Input: part model. Units: mm. Frame: model coordinates. A direction names the side the tool comes from. Round coordinates to 2 decimals unless told otherwise and drop trailing zeros. Loops run counter-clockwise (first coordinate to the right, second up) from the corner with the lowest first, then second, coordinate; pieces in that order, holes last. Notation, with made-up numbers: (88.25, 65.25) -> (138.25, 65.25) arc R15 ccw to (138.25, 84.25) -> close; hole circle Ø7 at (53, 44.25). An arc over 180 degrees is marked (long way). One line per question, with ' | ' between items. Start each with the question number.
Q1. Cut plane A-A on x = 4. Return loops of the section in (y, z).
Q2. Contact query for flat-ended pins moving along their axis: P1, Ø1.6, axis at x = 55, y = -18, coming from the -Z side; P2, Ø5, axis at x = 1.5, y = -9, coming from the -Z side; P3, Ø5, axis at x = 63.5, y = -1.5, coming from the +Z side. Output: stop coordinate, or through.
Q3. Cut plane C-C on x = 31. Return loops of the section in (y, z).
Q4. Cut plane D-D on y = 4. Return loops of the section in (x, z).
Q5. Cut plane B-B on x = 65. Return loops of the section in (y, z), and give its area (3 significant figures).
Q6. Material intervals for L1, parallel to Z at x = 80, y = 15.75; L2, parallel to Y at x = 11, z = -10; L3, parallel to Z at x = 48.5, y = 14, sorted ascending.
Q7. Access query for faces 1 (the face through (94, 18, 7)), 2 (the face through (26, 16, -17)), 3 (the face through (90.959, -0.224, -57.393)). Directions: +Z, -Z, +X, -X, +Y, -Y. A direction counts if a zero-diameter tool reaches every point of the face in a straight line with its end or side. Return the directions, or none.
Q8. Mould query, pull axis Y, two halves, no side actions, for faces 4 (the face through (35.9, 12.4, 9)), 5 (the face through (74, 19, 5)), 6 (the face through (93.14, -17.99, -2.1)). Classes: pulls with the +Y half, pulls with the -Y half, needs draft (parallel to the pull), parting line crosses it, or undercut.
from build123d import *

# Parameters (mm, degrees)
F1_DEPTH  = 16
F2_W      = 70
F2_H      = 3
F3_DEPTH  = 2
F4_W      = 50
F4_H      = 14
F5_DEPTH  = 2
F6_R      = 1
F9_DEPTH  = 2
F11_DEPTH = 38.001
F13_D     = 4
F14_R     = 3
F14_R_2   = 2
F15_DEPTH = 5
F16_R     = 3


# Not quite as in the source:
# - a pattern or mirror of a feature is missing from the dataset's text; its kind, count and spacing are read off the source's solid


with BuildPart() as f1:
    # F0 (on Front) → F1 (new body)
    with BuildSketch(Plane.XZ):
        with BuildLine():
            Line((94, 11), (0, 11))
            ThreePointArc((0, 11), (-11, 0), (0, -11))
            Line((0, -11), (19, -11))
            ThreePointArc((19, -11), (21.7681124643, -11.8361612201), (23.6103896104, -14.064978646))
            ThreePointArc((23.6103896104, -14.064978646), (47.9223026847, -44.6255578719), (84.6125434697, -57.9988278946))
            ThreePointArc((84.6125434697, -57.9988278946), (90.1511361286, -59.2227601314), (94.7495356371, -62.543714922))
            Line((94.7495356371, -62.543714922), (96.0448662588, -61))
            ThreePointArc((96.0448662588, -61), (90.8779784788, -57.357163598), (84.7034264019, -56))
            ThreePointArc((84.7034264019, -56), (49.0672193413, -42.9854179344), (25.4545454545, -13.2909701044))
            ThreePointArc((25.4545454545, -13.2909701044), (22.87535745, -10.1706257081), (19, -9))
            Line((19, -9), (0, -9))
            ThreePointArc((0, -9), (-9, 0), (0, 9))
            Line((0, 9), (94, 9))
            Line((94, 9), (94, 11))
        make_face()
    extrude(amount=F1_DEPTH)

    # F2 (on face) → F3 (join)
    with BuildSketch(Plane.XY.offset(11)):
        with Locations((59, -17.5)):
            Rectangle(F2_W, F2_H)
    extrude(amount=-F3_DEPTH)

    # F4 (on face) → F5 (join)
    with BuildSketch(Plane.XZ.offset(19)):
        with Locations((69, 4)):
            Rectangle(F4_W, F4_H)
    extrude(amount=-F5_DEPTH)

    # F6
    f6_edges = [f1.edges().sort_by_distance(p)[0] for p in [
        (59, -19, 11),
    ]]
    fillet(f6_edges, radius=F6_R)

    # F7: F1 across plane


with BuildPart() as f1_1:
    add(f1.part)
    add(f1.part.mirror(Plane.XZ))

    # F8 (on face) → F9 (cut)
    with BuildSketch(Plane.XY.offset(11)):
        with BuildLine():
            Line((94, 12), (34, 12))
            ThreePointArc((34, 12), (22, 0), (34, -12))
            Line((34, -12), (94, -12))
            Line((94, -12), (94, 12))
        make_face()
    extrude(amount=-F9_DEPTH, mode=Mode.SUBTRACT)

    # F10 (on face) → F11 (cut, through all)
    with BuildSketch(Plane.XZ.offset(19)):
        with BuildLine():
            ThreePointArc((50, 5), (47, 2), (50, -1))
            Line((50, -1), (70, -1))
            ThreePointArc((70, -1), (73, 2), (70, 5))
            Line((70, 5), (50, 5))
        make_face()
    extrude(amount=-F11_DEPTH, mode=Mode.SUBTRACT)

    # F13 (through all)
    with Locations(Plane.XZ.offset(19)):
        with Locations((80, 3)):
            Hole(F13_D / 2)

    # F14 (on face) → F15 (join)
    with BuildSketch(Plane(origin=(0, -17, 0), x_dir=(-1, 0, 0), z_dir=(0, 1, 0))):
        with Locations((-80, 3)):
            Circle(F14_R)
        with Locations((-80, 3)):
            Circle(F14_R_2, mode=Mode.SUBTRACT)
    f15 = extrude(amount=F15_DEPTH)

    # F15_copies: F15 across plane
    add(f15.mirror(Plane.ZX))

    # F16
    f16_edges = [f1_1.edges().sort_by_distance(p)[0] for p in [
        (94, 18, -3),
        (44, 18, -3),
        (44, -18, -3),
        (94, -18, -3),
    ]]
    fillet(f16_edges, radius=F16_R)


solid = f1_1.part
Results:
1) outline: (-16, -11) -> (16, -11) -> (16, -9) -> (-16, -9) -> close; (-16, 9) -> (16, 9) -> (16, 11) -> (-16, 11) -> close
2) P1: z = -3 | P2: z = -11 | P3: z = -49.91
3) outline: (-19, 9) -> (-11.62, 9) -> (-11.62, 11) -> (-18, 11) arc R1 ccw to (-19, 10) -> close; (-16, -27.47) -> (16, -27.47) -> (16, -23.87) -> (-16, -23.87) -> close; (11.62, 9) -> (19, 9) -> (19, 10) arc R1 ccw to (18, 11) -> (11.62, 11) -> close
4) outline: (0, -11) -> (19, -11) arc R5 cw to (23.61, -14.06) arc R72 ccw to (84.61, -58) arc R14 cw to (94.75, -62.54) -> (96.04, -61) arc R16 ccw to (84.7, -56) arc R70 cw to (25.45, -13.29) arc R7 ccw to (19, -9) -> (0, -9) arc R9 cw to (0, 9) -> (22.69, 9) -> (22.69, 11) -> (0, 11) arc R11 ccw to start
5) outline: (-19, -3) -> (-17, -3) -> (-17, -1) -> (-19, -1) -> close; (-19, 5) -> (-17, 5) -> (-17, 9) -> (-12, 9) -> (-12, 11) -> (-18, 11) arc R1 ccw to (-19, 10) -> close; (-16, -53.72) -> (16, -53.72) -> (16, -51.58) -> (-16, -51.58) -> close; (12, 9) -> (17, 9) -> (17, 5) -> (19, 5) -> (19, 10) arc R1 ccw to (18, 11) -> (12, 11) -> close; (17, -3) -> (19, -3) -> (19, -1) -> (17, -1) -> close | area: 120 mm^2
6) L1: -57.5 to -55.48, 0 to 1, 5 to 6, 9 to 11 | L2: -16 to 16 | L3: -45.04 to -42.57, 9 to 11
7) face 1: +Z, +X, +Y, -Y | face 2: -Z, -X, +Y | face 3: +X, +Y, -Y
8) face 4: undercut | face 5: pulls with the +Y half | face 6: needs draft
